Work out the finished part from the listing and answer in its coordinate system (mm). A direction names the side the tool comes from. Round coordinates to 2 decimals unless told otherwise and drop trailing zeros. Use CSV: the item, a comma, the result in double quotes. Start each with the question number.
Autodesk Inventor part; units mm, degrees
ref_plane "YZ Plane" through (0, 0, 0) normal (1, 0, 0) x (0, 1, 0)
ref_plane "XZ Plane" through (0, 0, 0) normal (0, 1, 0) x (-1, 0, 0)
ref_plane "XY Plane" through (0, 0, 0) normal (0, 0, 1) x (1, 0, 0)
sketch "スケッチ1" plane through (0, 0, 0) normal (0, 1, 0) x (-1, 0, 0)
  line L0 (30, 0) -> (-30, 0)
  line L1 (-30, 0) -> (-30, -45)
  line L2 (-30, -45) -> (30, -45)
  line L3 (30, -45) -> (30, 0)
  line L4 (37, 0) -> (30, 0)
  line L5 (30, 0) -> (30, -45)
  line L6 (30, -45) -> (37, -45)
  line L7 (37, -45) -> (37, 0)
  line L8 (-30, 0) -> (-37, 0)
  line L9 (-37, 0) -> (-37, -45)
  line L10 (-37, -45) -> (-30, -45)
  line L11 (-30, -45) -> (-30, 0)
  line L12 (37, 0) -> (35, 0)
  line L13 (35, 0) -> (35, -45) construction
  line L14 (35, -45) -> (37, -45)
  line L15 (37, -45) -> (37, 0)
  line L16 (-37, 0) -> (-35, 0)
  line L17 (-35, 0) -> (-35, -45) construction
  line L18 (-35, -45) -> (-37, -45)
  line L19 (-37, -45) -> (-37, 0)
  circle A0 centre (35, -5) radius 0.8
  circle A1 centre (35, -40) radius 0.8
  circle A2 centre (-35, -5) radius 0.8
  circle A3 centre (-35, -40) radius 0.8
  circle A4 centre (-35, -22.5) radius 0.8
  circle A5 centre (35, -22.5) radius 0.8
  point P0 (0, 0)
  point P1 (0, 0)
  point P2 (30, 0)
  dimension "d0" = 60
  dimension "d1" = 45
  dimension "d4" = 7
  dimension "d5" = 2
  dimension "d6" = 2
  dimension "d7" = 1.6
  dimension "d8" = 1.6
  dimension "d9" = 1.6
  dimension "d10" = 1.6
  dimension "d11" = 5
  dimension "d12" = 5
  dimension "d13" = 1.6
  dimension "d14" = 1.6
extrude "押し出し1" add sketch "スケッチ1" along normal blind 1.5
sketch "スケッチ2" plane through (0, 1.5, 0) normal (0, 1, 0) x (1, 0, 0)
  circle A0 centre (-35, 40) radius 0.8
  circle A1 centre (35, 5) radius 0.8
  line L0 (-35, 40) -> (35, 40)
  line L1 (35, 40) -> (35, 5)
  line L2 (35, 5) -> (-35, 5)
  line L3 (-35, 5) -> (-35, 40)
  line L4 (-32, 40) -> (32, 40)
  line L5 (32, 40) -> (32, 5)
  line L6 (32, 5) -> (-32, 5)
  line L7 (-32, 5) -> (-32, 40)
  line L8 (-26.2857, 40) -> (-22.2857, 40)
  line L9 (-22.2857, 40) -> (-22.2857, 5)
  line L10 (-22.2857, 5) -> (-26.2857, 5)
  line L11 (-26.2857, 5) -> (-26.2857, 40)
  line L12 (-16.5714, 40) -> (-12.5714, 40)
  line L13 (-12.5714, 40) -> (-12.5714, 5)
  line L14 (-12.5714, 5) -> (-16.5714, 5)
  line L15 (-16.5714, 5) -> (-16.5714, 40)
  line L16 (-6.8571, 40) -> (-2.8571, 40)
  line L17 (-2.8571, 40) -> (-2.8571, 5)
  line L18 (-2.8571, 5) -> (-6.8571, 5)
  line L19 (-6.8571, 5) -> (-6.8571, 40)
  line L20 (2.8571, 40) -> (6.8571, 40)
  line L21 (6.8571, 40) -> (6.8571, 5)
  line L22 (6.8571, 5) -> (2.8571, 5)
  line L23 (2.8571, 5) -> (2.8571, 40)
  line L24 (12.5714, 40) -> (16.5714, 40)
  line L25 (16.5714, 40) -> (16.5714, 5)
  line L26 (16.5714, 5) -> (12.5714, 5)
  line L27 (12.5714, 5) -> (12.5714, 40)
  line L28 (22.2857, 40) -> (26.2857, 40)
  line L29 (26.2857, 40) -> (26.2857, 5)
  line L30 (26.2857, 5) -> (22.2857, 5)
  line L31 (22.2857, 5) -> (22.2857, 40)
  point P0 (0, 0)
  point P1 (32, 40)
  point P2 (6.8571, 5)
  dimension "d16" = 3
  dimension "d17" = 3
  dimension "d18" = 4
  dimension "d19" = 5.7143
  dimension "d20" = 5.7143
  dimension "d21" = 5.7143
  dimension "d22" = 5.7143
  dimension "d23" = 5.7143
  dimension "d24" = 5.7143
  dimension "d25" = 5.7143
extrude "押し出し2" cut sketch "スケッチ2" against normal through all contours L0 L11 L2 L7 | L0 L15 L2 L9 | L0 L19 L2 L13 | L0 L23 L2 L17 | L0 L27 L2 L21 | L0 L31 L2 L25 | L0 L5 L2 L29
fillet "フィレット1" radius 2 32 edges at (-37, 0.75, 0) (-37, 0.75, -45) (37, 0.75, 0) (37, 0.75, -45) (-32, 0.75, -40) (-22.2857, 0.75, -40) (-12.5714, 0.75, -40) (-2.8571, 0.75, -40) (6.8571, 0.75, -40) (16.5714, 0.75, -40) (26.2857, 0.75, -40) (32, 0.75, -40) (22.2857, 0.75, -40) (12.5714, 0.75, -40) (2.8571, 0.75, -40) (-6.8571, 0.75, -40) (-16.5714, 0.75, -40) (-26.2857, 0.75, -40) (-26.2857, 0.75, -5) (-16.5714, 0.75, -5) (-6.8571, 0.75, -5) (2.8571, 0.75, -5) (12.5714, 0.75, -5) (22.2857, 0.75, -5) (32, 0.75, -5) (-32, 0.75, -5) (-22.2857, 0.75, -5) (-12.5714, 0.75, -5) (-2.8571, 0.75, -5) (6.8571, 0.75, -5) (16.5714, 0.75, -5) (26.2857, 0.75, -5)
equation "\"d19\" = d25"
equation "\"d20\" = d25"
equation "\"d21\" = d25"
equation "\"d22\" = d25"
equation "\"d23\" = d25"
equation "\"d24\" = d25"
properties part number "chest_cover_top"
Item 1: The mould has two halves that part along Z. Classify faces 3 (the flat face through (-16, 0, -22)), 4 (the cylindrical face through (-36.4, 0.76, -44.43)), 5 (the cylindrical face through (21.684, 0.74, -39.43)): pulls with the +Z half, pulls with the -Z half, needs draft (parallel to the pull), parting line crosses it, or undercut.
Item 2: This flat-tipped pin is pushed along its axis until it touches: pin 1 Ø1.3 at (x, z) = (-35, -5) entering from -Y. Where does it stop, or does it pass through?
Item 3: Which of the six approach directions +Z, -Z, +X, -X, +Y, -Y give full straight-line access (tool end or side, diameter ignored) to faces 1 (the flat face through (37, 1, -22)), 2 (the flat face through (26.286, 1, -23))?
Item 4: A cutting plane is placed at A-A (z = -26). State how many separate pieces and enclosed holes the cut face has, plus the area to 3 significant figures.
Item 5: Find the intervals of material crossed by probe 1 along Z at (x, y) = (35, 0.6), in increasing order. Write a range as [from, to].
Result sheet:
1,face 3,"needs draft"
1,face 4,"pulls with the -Z half"
1,face 5,"undercut"
2,pin 1,"through"
3,face 1,"+Z, -Z, +X, +Y, -Y"
3,face 2,"+Y, -Y"
4,separate pieces,"8"
4,enclosed holes,"0"
4,area,"51.0 mm^2"
5,probe 1,"[-45, -40.8], [-39.2, -23.3], [-21.7, -5.8], [-4.2, 0]"
